The listing builds one solid part. Answer for the finished solid, in the listing's coordinates (mm). Face numbers are marked on the shaded views. A direction names the side the tool comes from. Round coordinates to 2 decimals unless told otherwise and drop trailing zeros. Order: outer loops, then holes, each group sorted by start corner. A loop starts at its lowest first (then second) coordinate and runs counter-clockwise, first axis right, second up. Notation, with made-up numbers: (36, -1) -> (53, -1) arc R14 ccw to (53, 4) -> close; hole circle Ø4 at (39, 41.25). An arc over 180 degrees is marked (long way). Answer in a Markdown table with one row per item. Add a question column.
```python
from build123d import *

# Parameters (mm, degrees)
BOSS_EXTRUDE2_DEPTH = 2
CHAMFER1_SIZE       = 1
CHAMFER1_SIZE2      = 5


with BuildPart() as part:
    # Sketch2 → Revolve1 (revolve)
    with BuildSketch(Plane.XY, mode=Mode.PRIVATE) as revolve1_sk:
        Polygon((0, 0), (18.75, 0), (18.75, 10), (24, 14.630064794), (24, 17.630064794), (0, 17.630064794), align=None)
    revolve(revolve1_sk.sketch.rotate(Axis((0, 17.630064794, 0), (0, -1, 0)), 180), axis=Axis((0, 17.630064794, 0), (0, -1, 0)))

    # Sketch3 → Boss-Extrude2 (add)
    # profile 1 of 4: a face of its own
    with BuildSketch(Plane(origin=(0, 17.630064794, 0), x_dir=(1, 0, 0), z_dir=(0, 1, 0))):
        with BuildLine():
            add(Edge.make_bspline(
                [(0, -17.615132118), (9.89752, -17.615132118), (17.92, -9.592652118), (17.92, 0.304867882)],
                knots=[0, 0, 0, 0, 1, 1, 1, 1], degree=3))
            add(Edge.make_bspline(
                [(17.92, 0.304867882), (17.92, 10.202387882), (9.89752, 18.224867882), (0, 18.224867882)],
                knots=[0, 0, 0, 0, 1, 1, 1, 1], degree=3))
            add(Edge.make_bspline(
                [(0, 18.224867882), (-9.89752, 18.224867882), (-17.92, 10.202387882), (-17.92, 0.304867882)],
                knots=[0, 0, 0, 0, 1, 1, 1, 1], degree=3))
            add(Edge.make_bspline(
                [(-17.92, 0.304867882), (-17.92, -9.592652118), (-9.89752, -17.615132118), (0, -17.615132118)],
                knots=[0, 0, 0, 0, 1, 1, 1, 1], degree=3))
        make_face()
        with BuildLine():
            add(Edge.make_bspline(
                [(0, -15.055132118), (-8.47, -15.055132118), (-15.36, -8.165132118), (-15.36, 0.304867882)],
                knots=[0, 0, 0, 0, 1, 1, 1, 1], degree=3))
            add(Edge.make_bspline(
                [(-15.36, 0.304867882), (-15.36, 8.774867882), (-8.47, 15.664867882), (0, 15.664867882)],
                knots=[0, 0, 0, 0, 1, 1, 1, 1], degree=3))
            add(Edge.make_bspline(
                [(0, 15.664867882), (8.47, 15.664867882), (15.36, 8.774867882), (15.36, 0.304867882)],
                knots=[0, 0, 0, 0, 1, 1, 1, 1], degree=3))
            add(Edge.make_bspline(
                [(15.36, 0.304867882), (15.36, -8.165132118), (8.47, -15.055132118), (0, -15.055132118)],
                knots=[0, 0, 0, 0, 1, 1, 1, 1], degree=3))
        make_face(mode=Mode.SUBTRACT)
    # profile 2 of 4: a face of its own
    with BuildSketch(Plane(origin=(0, 17.630064794, 0), x_dir=(1, 0, 0), z_dir=(0, 1, 0))):
        with BuildLine():
            add(Edge.make_bspline(
                [(5.12, 1.584867882), (6.53496, 1.584867882), (7.68, 3.302387882), (7.68, 5.424867882)],
                knots=[0, 0, 0, 0, 1, 1, 1, 1], degree=3))
            add(Edge.make_bspline(
                [(7.68, 5.424867882), (7.68, 7.544867882), (6.53504, 9.264867882), (5.12, 9.264867882)],
                knots=[0, 0, 0, 0, 1, 1, 1, 1], degree=3))
            add(Edge.make_bspline(
                [(5.12, 9.264867882), (3.70496, 9.264867882), (2.56, 7.544867882), (2.56, 5.424867882)],
                knots=[0, 0, 0, 0, 1, 1, 1, 1], degree=3))
            add(Edge.make_bspline(
                [(2.56, 5.424867882), (2.56, 3.302387882), (3.70504, 1.584867882), (5.12, 1.584867882)],
                knots=[0, 0, 0, 0, 1, 1, 1, 1], degree=3))
        make_face()
    # profile 3 of 4: a face of its own
    with BuildSketch(Plane(origin=(0, 17.630064794, 0), x_dir=(1, 0, 0), z_dir=(0, 1, 0))):
        with BuildLine():
            add(Edge.make_bspline(
                [(-5.12, 1.584867882), (-3.70504, 1.584867882), (-2.56, 3.302387882), (-2.56, 5.424867882)],
                knots=[0, 0, 0, 0, 1, 1, 1, 1], degree=3))
            add(Edge.make_bspline(
                [(-2.56, 5.424867882), (-2.56, 7.544867882), (-3.70496, 9.264867882), (-5.12, 9.264867882)],
                knots=[0, 0, 0, 0, 1, 1, 1, 1], degree=3))
            add(Edge.make_bspline(
                [(-5.12, 9.264867882), (-6.53504, 9.264867882), (-7.68, 7.544867882), (-7.68, 5.424867882)],
                knots=[0, 0, 0, 0, 1, 1, 1, 1], degree=3))
            add(Edge.make_bspline(
                [(-7.68, 5.424867882), (-7.68, 3.302387882), (-6.53496, 1.584867882), (-5.12, 1.584867882)],
                knots=[0, 0, 0, 0, 1, 1, 1, 1], degree=3))
        make_face()
    # profile 4 of 4: a face of its own
    with BuildSketch(Plane(origin=(0, 17.630064794, 0), x_dir=(1, 0, 0), z_dir=(0, 1, 0))):
        with BuildLine():
            add(Edge.make_bspline(
                [(0, -11.215132118), (5.27496, -11.215132118), (9.99, -7.677612118), (11.47, -2.612652118)],
                knots=[0, 0, 0, 0, 1, 1, 1, 1], degree=3))
            add(Edge.make_bspline(
                [(11.47, -2.612652118), (11.66752, -1.935132118), (11.27752, -1.225132118), (10.59752, -1.025132118)],
                knots=[0, 0, 0, 0, 1, 1, 1, 1], degree=3))
            add(Edge.make_bspline(
                [(10.59752, -1.025132118), (9.92, -0.822652118), (9.21, -1.220172118), (9.01, -1.895132118)],
                knots=[0, 0, 0, 0, 1, 1, 1, 1], degree=3))
            add(Edge.make_bspline(
                [(9.01, -1.895132118), (7.85, -5.875132118), (4.14504, -8.655132118), (0, -8.655132118)],
                knots=[0, 0, 0, 0, 1, 1, 1, 1], degree=3))
            add(Edge.make_bspline(
                [(0, -8.655132118), (-4.14504, -8.655132118), (-7.85, -5.875132118), (-9.01128, -1.895132118)],
                knots=[0, 0, 0, 0, 1, 1, 1, 1], degree=3))
            add(Edge.make_bspline(
                [(-9.01128, -1.895132118), (-9.2088, -1.220092118), (-9.91128, -0.822652118), (-10.5988, -1.025132118)],
                knots=[0, 0, 0, 0, 1, 1, 1, 1], degree=3))
            add(Edge.make_bspline(
                [(-10.5988, -1.025132118), (-11.27752, -1.225132118), (-11.66632, -1.935132118), (-11.4688, -2.612652118)],
                knots=[0, 0, 0, 0, 1, 1, 1, 1], degree=3))
            add(Edge.make_bspline(
                [(-11.4688, -2.612652118), (-9.99128, -7.677612118), (-5.27496, -11.215132118), (0, -11.215132118)],
                knots=[0, 0, 0, 0, 1, 1, 1, 1], degree=3))
        make_face()
    extrude(amount=BOSS_EXTRUDE2_DEPTH)

    # Chamfer1
    chamfer1_edges = [part.edges().sort_by_distance(p)[0] for p in [
        (18.75, 0, 0),
    ]]
    chamfer1_side = [part.faces().sort_by_distance(p)[0] for p in [
        (0, 0, 0),
    ]]
    chamfer(chamfer1_edges, length=CHAMFER1_SIZE, length2=CHAMFER1_SIZE2, reference=chamfer1_side[0])


solid = part.part
```
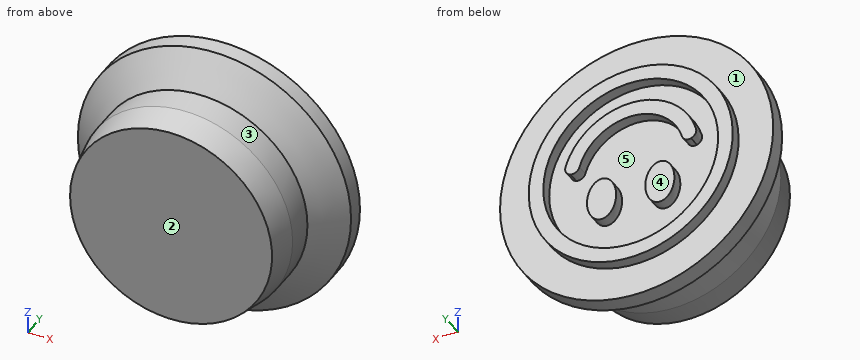
Item 1: For a pull along Z with two mould halves and no side action, classify the marked faces 3, 4 and 5 as released by +Z, released by -Z, zero draft, split by the parting line, or undercut.
Item 2: The part is cut by section A-A, the plane y = 4. Give the vertices of the cut face in (x, z), and give its area (3 significant figures).
Item 3: The part is cut by section B-B, the plane y = 12.5. Give the vertices of the cut face in (x, z), and give its area (3 significant figures).
Item 4: Flat-ended cylindrical pins translate along their axes: P1, Ø4, axis at y = 9.5, z = -13, coming from the -X side; P2, Ø10, axis at x = -11.5, y = 16, coming from the -Z side; P3, Ø5, axis at y = 12.5, z = 1, coming from the +X side; P4, Ø8, axis at x = 6, y = 5.5, coming from the +Z side. Find the tip coordinate at first contact, or state that the pin passes through.
Item 5: Find the intervals of material crossed by probe 1 along Z at (x, y) = (2, 18.5); probe 2 along X at (y, z) = (17.75, -4.5); probe 3 along Y at (x, z) = (-11, -1.5), in increasing order. Write a range as [from, to].
Item 6: A tool of negligible diameter and unlimited length cuts with its end or side. For the marked faces 1 and 2, from which of +Z, -Z, +X, -X, +Y, -Y can it reach the whole face along a straight path? Write none if from no direction.
Resolved:
| question | item | result |
|---|---|---|
| 1 | face 3 | split by the parting line |
| 1 | face 4 | zero draft |
| 1 | face 5 | undercut |
| 2 | outline | circle Ø37.1 at (0, 0) |
| 2 | area | 1,080 mm2 |
| 3 | outline | circle Ø43.17 at (0, 0) |
| 3 | area | 1,460 mm2 |
| 4 | P1 | x = -16.19 |
| 4 | P2 | z = -23.1 |
| 4 | P3 | x = 24 |
| 4 | P4 | z = 18.64 |
| 5 | probe 1 | [-18.11, -15.54], [8.44, 11.04], [14.93, 17.5] |
| 5 | probe 2 | [-17.43, -14.78], [-7.61, -2.63], [2.63, 7.61], [14.78, 17.43] |
| 5 | probe 3 | [0, 17.63] |
| 6 | face 1 | +Y |
| 6 | face 2 | +Z, -Z, +X, -X, -Y |
